Could you check a few things on this model? Use its own coordinates, in mm. A direction names the side the tool comes from. Round coordinates to 2 decimals unless told otherwise and drop trailing zeros. Loops run counter-clockwise (first coordinate to the right, second up) from the corner with the lowest first, then second, coordinate; pieces in that order, holes last.
from build123d import *

# Parameters (mm, degrees)
PAD_DEPTH       = 1200
CHAMFER_SIZE    = 17
SKETCH001_W     = 382.5
SKETCH001_H     = 42.5
SKETCH001_H_2   = 40
POCKET_DEPTH    = 144
SKETCH002_W     = 100
SKETCH002_H     = 382.5
POCKET001_DEPTH = 800
CHAMFER001_SIZE = 7
CHAMFER002_SIZE = 7


with BuildPart() as part:
    # Sketch → Pad (new body)
    with BuildSketch(Plane.YZ):
        Polygon((800, 0), (800, 144), (655, 144), (655, 132), (612.5, 132), (612.5, 144), (512.5, 144), (512.5, 132), (472.5, 132), (472.5, 144), (327.5, 144), (327.5, 132), (287.5, 132), (287.5, 144), (187.5, 144), (187.5, 132), (145, 132), (145, 144), (0, 144), (0, 0), (100, 0), (100, 100), (327.5, 100), (327.5, 0), (472.5, 0), (472.5, 100), (700, 100), (700, 0), align=None)
    extrude(amount=PAD_DEPTH)

    # Chamfer
    chamfer_edges = [part.edges().sort_by_distance(p)[0] for p in [
        (1200, 0, 72),
        (0, 0, 72),
        (0, 800, 72),
        (1200, 800, 72),
    ]]
    chamfer(chamfer_edges, length=CHAMFER_SIZE)

    # Sketch001 → Pocket (cut)
    with BuildSketch(Plane.XY):
        with Locations((336.25, 166.25)):
            Rectangle(SKETCH001_W, SKETCH001_H)
        with Locations((863.75, 166.25)):
            Rectangle(SKETCH001_W, SKETCH001_H)
        with Locations((336.25, 307.5)):
            Rectangle(SKETCH001_W, SKETCH001_H_2)
        with Locations((863.75, 307.5)):
            Rectangle(SKETCH001_W, SKETCH001_H_2)
        with Locations((336.25, 492.5)):
            Rectangle(SKETCH001_W, SKETCH001_H_2)
        with Locations((863.75, 492.5)):
            Rectangle(SKETCH001_W, SKETCH001_H_2)
        with Locations((336.25, 633.75)):
            Rectangle(SKETCH001_W, SKETCH001_H)
        with Locations((863.75, 633.75)):
            Rectangle(SKETCH001_W, SKETCH001_H)
    extrude(amount=POCKET_DEPTH, mode=Mode.SUBTRACT)

    # Sketch002 (on Face2 of Pocket) → Pocket001 (cut)
    with BuildSketch(Plane.ZX.offset(800)):
        with Locations((72, 863.75)):
            Rectangle(SKETCH002_W, SKETCH002_H)
        with Locations((72, 336.25)):
            Rectangle(SKETCH002_W, SKETCH002_H)
    extrude(amount=-POCKET001_DEPTH, mode=Mode.SUBTRACT)

    # Chamfer001
    chamfer001_edges = [part.edges().sort_by_distance(p)[0] for p in [
        (863.75, 0, 22),
        (336.25, 0, 22),
        (863.75, 0, 122),
        (336.25, 0, 122),
    ]]
    chamfer(chamfer001_edges, length=CHAMFER001_SIZE)

    # Chamfer002
    chamfer002_edges = [part.edges().sort_by_distance(p)[0] for p in [
        (863.75, 800, 22),
        (863.75, 800, 122),
        (336.25, 800, 122),
        (336.25, 800, 22),
    ]]
    chamfer(chamfer002_edges, length=CHAMFER002_SIZE)


solid = part.part
Item 1: If we section it at C-C, the plane y = 161: Please give me the cut outline in (x, z), then the cut area to 3 significant figures.
Results list:
outline: (0, 100) - (145, 100) - (145, 132) - (0, 132) - close; (527.5, 100) - (672.5, 100) - (672.5, 132) - (527.5, 132) - close; (1055, 100) - (1200, 100) - (1200, 132) - (1055, 132) - close
area: 13,900 mm2
Item 2: Will these pins go through, and if not, where does the flat tip stop? pin 1 (8 mm diameter, centred on y = 318, z = 120.5, fed in from -X); pin 2 (12 mm diameter, centred on y = 292, z = 93, fed in from -X); pin 3 (12 mm diameter, centred on x = 634, y = 496.5, fed in from +Z).
Results list:
pin 1: stops at x = 0
pin 2: passes through
pin 3: stops at z = 132
Item 3: If we section it at B-B, the plane x = 102.5: Please give me the cut outline in (y, z).
Results list:
outline: (0, 0) - (100, 0) - (100, 100) - (327.5, 100) - (327.5, 0) - (472.5, 0) - (472.5, 100) - (700, 100) - (700, 0) - (800, 0) - (800, 144) - (655, 144) - (655, 132) - (612.5, 132) - (612.5, 144) - (512.5, 144) - (512.5, 132) - (472.5, 132) - (472.5, 144) - (327.5, 144) - (327.5, 132) - (287.5, 132) - (287.5, 144) - (187.5, 144) - (187.5, 132) - (145, 132) - (145, 144) - (0, 144) - close
Item 4: If we section it at D-D, the plane z = 46: Count the separate pieces of the cut face and the enclosed holes in it, then the cut area to 3 significant figures.
Results list:
separate pieces: 9
enclosed holes: 0
area: 149,000 mm2
Item 5: We'd pull the mould along Z, two halves only. Please class faces 6 (the flat face through (334, 401, 22)), 7 (the flat face through (334, 401, 122)), 8 (the flat face through (0, 395, 89)), 9 (the flat face through (71, 308, 132)): released by +Z, released by -Z, zero draft, split by the parting line, or undercut.
Results list:
face 6: undercut
face 7: undercut
face 8: zero draft
face 9: released by +Z
Item 6: If I drill on line 1 along X through (y, z) = (764, 113.5); line 2 along Y through (x, z) = (565, 135); line 3 along Y through (x, z) = (650, 74), over which ranges is the centre line in solid material (lowest first)?
Results list:
line 1: x = 0 to 145, 527.5 to 672.5, 1055 to 1200
line 2: y = 0 to 145, 187.5 to 287.5, 327.5 to 472.5, 512.5 to 612.5, 655 to 800
line 3: y = 0 to 100, 327.5 to 472.5, 700 to 800
Item 7: For faces 1 (the flat face through (861, 563, 122)), 2 (the flat face through (1126, 308, 132)), 3 (the flat face through (592, 0, 73)), 4 (the flat face through (71, 585, 100)), 5 (the flat face through (592, 145, 133)), which set-ups out of +Z, -Z, +X, -X, +Y, -Y let a thin tool reach every point of the face, with its end or its side?
Results list:
face 1: -Z, +Y, -Y
face 2: +Z, +X, -X
face 3: +Z, -Z, +X, -X, -Y
face 4: -Z, +X, -X
face 5: +Z
Item 8: If we section it at A-A, the plane y = 362: Please give me the cut outline in (x, z), then the cut area to 3 significant figures.
Results list:
outline: (0, 0) - (1200, 0) - (1200, 144) - (0, 144) - close; hole (145, 22) - (527.5, 22) - (527.5, 122) - (145, 122) - close; hole (672.5, 22) - (1055, 22) - (1055, 122) - (672.5, 122) - close
area: 96,300 mm2
